from build123d import *

# Parameters (mm, degrees)
BOSS_EXTRUDE1_DEPTH      = 2
BOSS_EXTRUDE1_DEPTH_BACK = 2
SKETCH1_R                = 5
SKETCH1_R_2              = 1.5
FILLET1_R                = 0.2
SKETCH2_R                = 4
SKETCH2_R_2              = 2.5
CUT_EXTRUDE1_DEPTH       = 0.1
CUT_EXTRUDE2_START       = -0.1
SKETCH3_R                = 4
SKETCH3_R_2              = 2.5
CUT_EXTRUDE2_DEPTH       = 0.1


with BuildPart() as part:
    # Sketch1 → Boss-Extrude1 (new, two sides: drawn at the far end of the back side and taken through both)
    with BuildSketch(Plane(origin=(0, 0, 0), x_dir=(0, 0, -1), z_dir=(1, 0, 0)).offset(-BOSS_EXTRUDE1_DEPTH_BACK)):
        Circle(SKETCH1_R)
        Circle(SKETCH1_R_2, mode=Mode.SUBTRACT)
    extrude(amount=BOSS_EXTRUDE1_DEPTH + BOSS_EXTRUDE1_DEPTH_BACK)

    # Fillet1
    fillet1_edges = [part.edges().sort_by_distance(p)[0] for p in [
        (-2, 0, 5),
        (-2, 0, 1.5),
        (2, 0, 5),
        (2, 0, 1.5),
    ]]
    fillet(fillet1_edges, radius=FILLET1_R)

    # Sketch2 → Cut-Extrude1 (cut)
    with BuildSketch(Plane(origin=(2, 0, 0), x_dir=(0, 0, -1), z_dir=(1, 0, 0))):
        Circle(SKETCH2_R)
        Circle(SKETCH2_R_2, mode=Mode.SUBTRACT)
    extrude(amount=-CUT_EXTRUDE1_DEPTH, mode=Mode.SUBTRACT)

    # Sketch3 → Cut-Extrude2 (cut)
    with BuildSketch(Plane.ZY.offset(2).offset(CUT_EXTRUDE2_START)):
        with Locations(Location((0, 0, 0), (0, 0, 180))):
            Circle(SKETCH3_R)
        with Locations(Location((0, 0, 0), (0, 0, 180))):
            Circle(SKETCH3_R_2, mode=Mode.SUBTRACT)
    extrude(amount=CUT_EXTRUDE2_DEPTH, mode=Mode.SUBTRACT)


solid = part.part
Can you work these out from the model? Positions are in its coordinate system, mm. A direction names the side the tool comes from. Coordinates: 2 decimals unless noted, no trailing zeros. Write each loop counter-clockwise with the first axis right and the second up, starting at its lowest first coordinate (ties: lowest second). Pieces come first, ordered by that corner, then holes. Notation, with made-up numbers: M 48,48 L 100,48 A25 cw 100,74 Z; hole C -5,30 d3. An arc over 180 degrees is marked long. Use one line per item in the form item = value.
Q1. I need wall thicknesses on line 1 along Y through (x, z) = (0.7, 0); line 2 along X through (y, z) = (-2.25, 3); line 3 along Y through (x, z) = (0.85, 1). Which ranges of each line are inside material? Lowest first, please. Write a range as from..to.
Model answer:
line_1 = -5..-1.5, 1.5..5
line_2 = -1.9..1.9
line_3 = -4.9..-1.12, 1.12..4.9
Q2. If we section it at C-C (x = 0.15): Write out the boundary of the cut face in (y, z).
Model answer:
outline = C 0,0 d10; hole C 0,0 d3
Q3. We'd pull the mould along Z, two halves only. Please class faces 3 (the flat face through (2, -2, -1)), 4 (the cylindrical face through (-0.03, -4.88, 1.08)), 5 (the flat face through (-1.9, -2, -2)): +Z half, -Z half, draft (parallel to the pull), parting line (faces both ways), or undercut.
Model answer:
face_3 = draft
face_4 = parting line
face_5 = undercut
Q4. For faces 1 (the flat face through (2, 4, 2)), 2 (the flat face through (1.9, 2, -2)), which set-ups out of +Z, -Z, +X, -X, +Y, -Y let a thin tool reach every point of the face, with its end or its side?
Model answer:
face_1 = +Z, -Z, +X, +Y, -Y
face_2 = +X
Q5. For P1, Ø1, axis at x = -1, y = 2.5, coming from the +Z side, with a flat end and sliding along its axis, tell me the tip position at first contact or that it passes through.
Model answer:
P1 = 4.58
